Autodesk Inventor part; units mm, degrees
sketch "Sketch1" plane through (0, 0, 0) normal (0, 1, 0) x (-1, 0, 0)
  line L0 (30, -30) -> (-30, -30)
  line L1 (-30, -30) -> (-30, 30)
  line L2 (-30, 30) -> (30, 30)
  line L3 (30, 30) -> (30, -30)
  line L4 (0, -42) -> (0, 42)
  line L5 (-42, 0) -> (42, 0)
  point P0 (0, 0)
  point P1 (0, -30)
  point P2 (30, 0)
  dimension "d0" = 60
  dimension "d1" = 60
extrude "Extrusion1" add sketch "Sketch1" along normal mid plane 10
sketch "Sketch2" plane through (0, -5, 0) normal (0, -1, 0) x (1, 0, 0)
  line L0 (-30, -30) -> (-30, 30)
  line L1 (-30, 5) -> (-22, 5)
  line L2 (-22, 5) -> (-22, -5)
  line L3 (-22, -5) -> (-30, -5)
  line L4 (-30, -5) -> (-30, 5)
  arc A0 (-22, -5) -> (-22, 5) centre (-22, 0) ccw
  line L5 (-53.2, 0) -> (53.2, 0)
  line L6 (-25, 5) -> (-25, -5)
  line L7 (0, -53.2) -> (0, 53.2)
  line L8 (-5, -30) -> (-5, -22)
  arc A1 (5, -22) -> (-5, -22) centre (0, -22) ccw
  line L9 (5, -22) -> (5, -30)
  line L10 (5, -30) -> (-5, -30)
  line L11 (-5, -25) -> (5, -25)
  line L12 (-5, -22) -> (5, -22)
  line L13 (30, -5) -> (22, -5)
  arc A2 (22, 5) -> (22, -5) centre (22, 0) ccw
  line L14 (22, 5) -> (30, 5)
  line L15 (30, 5) -> (30, -5)
  line L16 (25, -5) -> (25, 5)
  line L17 (22, -5) -> (22, 5)
  line L18 (5, 30) -> (5, 22)
  arc A3 (-5, 22) -> (5, 22) centre (0, 22) ccw
  line L19 (-5, 22) -> (-5, 30)
  line L20 (-5, 30) -> (5, 30)
  line L21 (5, 25) -> (-5, 25)
  line L22 (5, 22) -> (-5, 22)
  line L23 (30, -30) -> (-30, -30)
  line L24 (30, 30) -> (30, -30)
  line L25 (30, -30) -> (24.3431, -24.3431)
  line L26 (30, -30) -> (38, -30) construction
  line L27 (20.8076, -27.8787) -> (22.9289, -30)
  line L28 (27.8787, -20.8076) -> (30, -22.9289)
  line L29 (24.3431, -24.3431) -> (27.8787, -20.8076)
  line L30 (24.3431, -24.3431) -> (20.8076, -27.8787)
  line L31 (22.9289, -30) -> (30, -22.9289)
  line L32 (22.9289, -30) -> (30, -30)
  line L33 (30, -22.9289) -> (30, -30)
  arc A4 (27.8787, -20.8076) -> (20.8076, -27.8787) centre (24.3431, -24.3431) ccw
  line L34 (27.8787, 20.8076) -> (30, 22.9289)
  line L35 (24.3431, 24.3431) -> (27.8787, 20.8076)
  arc A5 (20.8076, 27.8787) -> (27.8787, 20.8076) centre (24.3431, 24.3431) ccw
  line L36 (24.3431, 24.3431) -> (20.8076, 27.8787)
  line L37 (20.8076, 27.8787) -> (22.9289, 30)
  line L38 (22.9289, 30) -> (30, 30)
  line L39 (30, 30) -> (24.3431, 24.3431)
  line L40 (30, 22.9289) -> (22.9289, 30)
  line L41 (30, 22.9289) -> (30, 30)
  line L42 (-20.8076, 27.8787) -> (-22.9289, 30)
  line L43 (-24.3431, 24.3431) -> (-20.8076, 27.8787)
  arc A6 (-27.8787, 20.8076) -> (-20.8076, 27.8787) centre (-24.3431, 24.3431) ccw
  line L44 (-24.3431, 24.3431) -> (-27.8787, 20.8076)
  line L45 (-27.8787, 20.8076) -> (-30, 22.9289)
  line L46 (-30, 22.9289) -> (-30, 30)
  line L47 (-30, 30) -> (-24.3431, 24.3431)
  line L48 (-22.9289, 30) -> (-30, 22.9289)
  line L49 (-22.9289, 30) -> (-30, 30)
  line L50 (-27.8787, -20.8076) -> (-30, -22.9289)
  line L51 (-24.3431, -24.3431) -> (-27.8787, -20.8076)
  arc A7 (-20.8076, -27.8787) -> (-27.8787, -20.8076) centre (-24.3431, -24.3431) ccw
  line L52 (-24.3431, -24.3431) -> (-20.8076, -27.8787)
  line L53 (-20.8076, -27.8787) -> (-22.9289, -30)
  line L54 (-22.9289, -30) -> (-30, -30)
  line L55 (-30, -30) -> (-24.3431, -24.3431)
  line L56 (-30, -22.9289) -> (-22.9289, -30)
  line L57 (-30, -22.9289) -> (-30, -30)
  point P0 (0, 0)
  point P1 (-30, 0)
  point P2 (0, -30)
  point P3 (30, 0)
  point P4 (0, 30)
  point P5 (-30, -5)
  point P6 (20.8076, -20.8076)
  point P7 (20.8076, 20.8076)
  point P8 (-20.8076, 20.8076)
  point P9 (-20.8076, -20.8076)
  dimension "d4" = 10
  dimension "d5" = 8
  dimension "d6" = 3
  dimension "d9" = 360
  dimension "d33" = 135
  dimension "d34" = 5
  dimension "d35" = 5
  dimension "d37" = 8
  dimension "d38" = 3
  dimension "d39" = 7.0711
  dimension "d45" = 5
  dimension "d48" = 360
extrude "Extrusion2" cut sketch "Sketch2" against normal blind 2 contours L0 L47 L48 | L40 L39 L24 | L55 L56 L23 | L0 L56 L55 | L0 L5 L6 L3 | L8 L11 L7 L10 | L0 L1 L6 L5 | L7 L11 L9 L10 | L31 L25 L23 | L49 L48 L47 | L25 L31 L24 | L13 L16 L5 L15 | L16 L14 L15 L5 | L21 L19 L20 L7 | L7 L20 L18 L21 | L39 L40 L38
extrude "Extrusion3" cut sketch "Sketch2" against normal blind 4 contours L48 L47 L44 L45 | A3 L22 L7 | L7 L22 A3 | L34 L35 L39 L40 | L50 L51 L55 L56 | L56 L55 L52 L53 | A7 L52 L51 | L6 L5 L2 L3 | L8 L12 L7 L11 | L6 L1 L2 L5 | L2 L5 A0 | A1 L7 L12 | L7 L12 L9 L11 | L2 A0 L5 | A1 L12 L7 | L27 L30 L25 L31 | L44 L43 A6 | L48 L42 L43 L47 | A4 L29 L30 | L25 L29 L28 L31 | A2 L17 L5 | L5 L17 A2 | L17 L14 L16 L5 | L5 L16 L13 L17 | L22 L19 L21 L7 | L7 L21 L18 L22 | A5 L36 L35 | L39 L36 L37 L40
sketch "Sketch3" plane through (0, 5, 0) normal (0, 1, 0) x (1, 0, 0)
  circle A0 centre (-25, 25) radius 2.5
  line L0 (30, 30) -> (-30, 30)
  line L1 (-30, 30) -> (-30, -30)
  line L2 (-42, 0) -> (42, 0)
  line L3 (0, 42) -> (0, -42)
  circle A1 centre (-25, 15) radius 2.5
  circle A2 centre (-25, 5) radius 2.5
  circle A3 centre (-25, -5) radius 2.5
  circle A4 centre (-25, -15) radius 2.5
  circle A5 centre (-15, 25) radius 2.5
  circle A6 centre (-15, 15) radius 2.5
  circle A7 centre (-15, 5) radius 2.5
  circle A8 centre (-15, -5) radius 2.5
  circle A9 centre (-15, -15) radius 2.5
  circle A10 centre (-5, 25) radius 2.5
  circle A11 centre (-5, 15) radius 2.5
  circle A12 centre (-5, 5) radius 2.5
  circle A13 centre (-5, -5) radius 2.5
  circle A14 centre (-5, -15) radius 2.5
  circle A15 centre (5, 25) radius 2.5
  circle A16 centre (5, 15) radius 2.5
  circle A17 centre (5, 5) radius 2.5
  circle A18 centre (5, -5) radius 2.5
  circle A19 centre (5, -15) radius 2.5
  circle A20 centre (15, 25) radius 2.5
  circle A21 centre (15, 15) radius 2.5
  circle A22 centre (15, 5) radius 2.5
  circle A23 centre (15, -5) radius 2.5
  circle A24 centre (15, -15) radius 2.5
  circle A25 centre (-25, -25) radius 2.5
  circle A26 centre (-15, -25) radius 2.5
  circle A27 centre (-5, -25) radius 2.5
  circle A28 centre (5, -25) radius 2.5
  circle A29 centre (15, -25) radius 2.5
  circle A30 centre (25, 25) radius 2.5
  circle A31 centre (25, 15) radius 2.5
  circle A32 centre (25, 5) radius 2.5
  circle A33 centre (25, -5) radius 2.5
  circle A34 centre (25, -15) radius 2.5
  circle A35 centre (25, -25) radius 2.5
  point P0 (0, 0)
  dimension "d15" = 5
  dimension "d16" = 5
  dimension "d17" = 5
  dimension "d20" = 10
  dimension "d23" = 10
extrude "Extrusion4" cut sketch "Sketch3" against normal blind 5 contours A0 | A1 | A2 | A3 | A4 | A5 | A6 | A7 | A8 | A9 | A10 | A11 | A12 | A13 | A14 | A15 | A16 | A17 | A18 | A19 | A20 | A21 | A22 | A23 | A24 | A25 | A26 | A27 | A28 | A29 | A30 | A31 | A32 | A33 | A34 | A35
properties part number "Tile"
Source: CAD feature listing. Evaluate the final solid. Frame: model axes, mm. A direction names the side the tool comes from. Coordinates: 2 decimals unless noted, no trailing zeros. Write each loop counter-clockwise with the first axis right and the second up, starting at its lowest first coordinate (ties: lowest second). Pieces come first, ordered by that corner, then holes. Notation, with made-up numbers: (66.5, 3) - (103.5, 3) arc R31 cw to (103.5, 42) - close; hole circle Ø1 at (-31.5, -11). An arc over 180 degrees is marked (long way). Answer as a JSON object with one key per item and string values.
Q1. Section query B-B, the plane x = 0. Output: boundary loops of the cut face in (y, z), plus the area to 3 significant figures.
Ans:
{"outline": "(-5, -17) - (-1, -17) - (-1, -25) - (-3, -25) - (-3, -30) - (5, -30) - (5, 30) - (-3, 30) - (-3, 25) - (-1, 25) - (-1, 17) - (-5, 17) - close", "area": "516 mm2"}
Q2. Section query C-C, the plane z = 15. Output: boundary loops of the cut face in (x, y).
Ans:
{"outline": "(-30, -5) - (30, -5) - (30, 5) - (27.5, 5) - (27.5, 0) - (22.5, 0) - (22.5, 5) - (17.5, 5) - (17.5, 0) - (12.5, 0) - (12.5, 5) - (7.5, 5) - (7.5, 0) - (2.5, 0) - (2.5, 5) - (-2.5, 5) - (-2.5, 0) - (-7.5, 0) - (-7.5, 5) - (-12.5, 5) - (-12.5, 0) - (-17.5, 0) - (-17.5, 5) - (-22.5, 5) - (-22.5, 0) - (-27.5, 0) - (-27.5, 5) - (-30, 5) - close"}
Q3. Draft query along Z for faces 1 (the flat face through (-25.1, -3.5, -5)), 2 (the cylindrical face through (-17, -3, 0)). Return one class per face: released by +Z, released by -Z, zero draft, split by the parting line, or undercut.
Ans:
{"face 1": "undercut", "face 2": "undercut"}
Q4. Set-up query: faces 3 (the cylindrical face through (20.886, -3.028, -20.731)), 4 (the flat face through (-15, 0, -25)). Return all of +Z, -Z, +X, -X, +Y, -Y with unobstructed straight access to the full face (end or side cutting, diameter ignored); none if empty.
Ans:
{"face 3": "-Y", "face 4": "+Y"}
Q5. Material intervals for line 1 (X direction, y = -2.5, z = 20.5); line 2 (Z direction, x = 21, y = -1.75); line 3 (Y direction, x = 5.5, z = -25), sorted ascending. Write a range as [from, to].
Ans:
{"line 1": "x = [-30, -27.54], [-21.14, -4.77], [4.77, 21.14], [27.54, 30]", "line 2": "z = [-30, -28.07], [-20.63, -4.9], [4.9, 20.63], [28.07, 30]", "line 3": "y = [-5, 0]"}
Q6. First-contact query: pin 1 Ø3 at (x, z) = (5, -5) entering from +Y; pin 2 Ø1.2 at (y, z) = (-4, 27) entering from -X; pin 3 Ø6.5 at (x, z) = (25, 25) entering from -Y. Flat tips, straight axial feed; report the tip coordinate or a pass-through.
Ans:
{"pin 1": "stops at y = 0", "pin 2": "stops at x = -20.55", "pin 3": "stops at y = -3"}
